from build123d import *

# Parameters (mm, degrees)
PAD_DEPTH       = 7
POCKET_DEPTH    = 10.001
SKETCH002_R     = 2
POCKET001_DEPTH = 7.001
FILLET_R        = 2


with BuildPart() as part:
    # Sketch → Pad (new body)
    with BuildSketch(Plane.XY):
        with BuildLine():
            Line((0, 0), (10, 0))
            Line((10, 0), (10, 17))
            ThreePointArc((10, 17), (5.000011, 22.000022), (0, 17.000022))
            Line((0, 17.000022), (0, 0))
        make_face()
    extrude(amount=PAD_DEPTH)

    # Sketch001 → Pocket (cut, through all)
    with BuildSketch(Plane.YZ.offset(10)):
        Polygon((10, 8), (23, 8), (23, 3.75), (10, 7), align=None)
    extrude(amount=-POCKET_DEPTH, mode=Mode.SUBTRACT)

    # Sketch002 → Pocket001 (cut, through all)
    with BuildSketch(Plane.XY.offset(7)):
        with Locations((5, 5)):
            Circle(SKETCH002_R)
    extrude(amount=-POCKET001_DEPTH, mode=Mode.SUBTRACT)

    # Fillet
    fillet_edges = [part.edges().sort_by_distance(p)[0] for p in [
        (0, 0, 3.5),
        (10, 0, 3.5),
    ]]
    fillet(fillet_edges, radius=FILLET_R)


solid = part.part
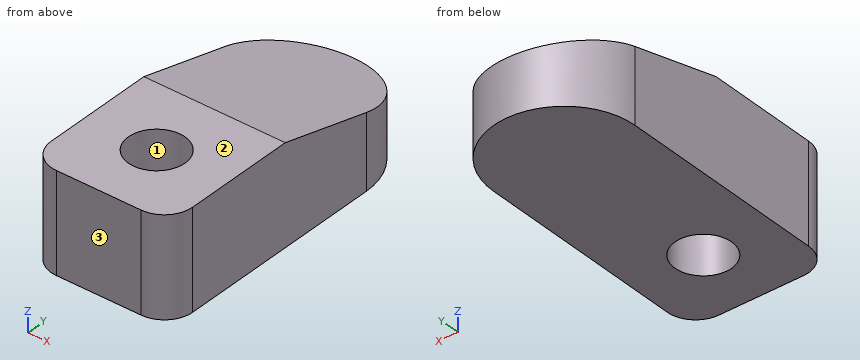
Can you work these out from the model? Positions are in its coordinate system, mm. Face numbers are marked on the shaded views. Coordinates: 2 decimals unless noted, no trailing zeros. Write each loop counter-clockwise with the first axis right and the second up, starting at its lowest first coordinate (ties: lowest second). Pieces come first, ordered by that corner, then holes. Notation, with made-up numbers: M 49.5,-17.5 L 64.5,-17.5 A26 ccw 64.5,10.5 Z; hole C 54.25,79.5 d1. An arc over 180 degrees is marked long. Use one line per item in the form item = value.
Q1. I need wall thicknesses on line 1 along Y through (x, z) = (5, 2.25); line 2 along Y through (x, z) = (8.75, 3); line 3 along Z through (x, y) = (2.5, 19). Which ranges of each line are inside material? Lowest first, please. Write a range as from..to.
Model answer:
line_1 = 0..3, 7..22
line_2 = 0.15..20.31
line_3 = 0..4.75
Q2. If we section it at D-D (z = 3.25): Write out the boundary of the cut face in (x, y), then the cut area to 3 significant figures.
Model answer:
outline = M 0,2 A2 ccw 2,0 L 8,0 A2 ccw 10,2 L 10,17 A5 ccw 0,17 Z; hole C 5,5 d4
area = 195 mm^2
Q3. For P1, Ø1.5, axis at x = 8, y = 15.5, coming from the +Z side, with a flat end and sliding along its axis, tell me the tip position at first contact or that it passes through.
Model answer:
P1 = 5.81
Q4. If we section it at B-B (z = 6): Write out the boundary of the cut face in (x, y), then the cut area to 3 significant figures.
Model answer:
outline = M 0,2 A2 ccw 2,0 L 8,0 A2 ccw 10,2 L 10,14 L 0,14 Z; hole C 5,5 d4
area = 126 mm^2
Q5. If we section it at A-A (x = 5): Write out the boundary of the cut face in (y, z), then the cut area to 3 significant figures.
Model answer:
outline = M 0,0 L 3,0 L 3,7 L 0,7 Z; M 7,0 L 22,0 L 22,4 L 10,7 L 7,7 Z
area = 108 mm^2
Q6. If we section it at C-C (y = 5): Write out the boundary of the cut face in (x, z), then the cut area to 3 significant figures.
Model answer:
outline = M 0,0 L 3,0 L 3,7 L 0,7 Z; M 7,0 L 10,0 L 10,7 L 7,7 Z
area = 42.0 mm^2
Q7. We'd pull the mould along Y, two halves only. Please class the marked faces 1, 2 and 3: +Y half, -Y half, draft (parallel to the pull), parting line (faces both ways), or undercut.
Model answer:
face_1 = undercut
face_2 = draft
face_3 = -Y half
